Autodesk Inventor part; units mm, degrees
ref_plane "YZ Plane" through (0, 0, 0) normal (1, 0, 0) x (0, 1, 0)
ref_plane "XZ Plane" through (0, 0, 0) normal (0, 1, 0) x (-1, 0, 0)
sketch "Sketch1" plane through (0, 0, 0) normal (0, 1, 0) x (-1, 0, 0)
  circle A0 centre (0, 0) radius 75
  dimension "d0" = 150
extrude "Extrusion1" add sketch "Sketch1" along normal blind 200
sketch "Sketch2" plane through (0, 200, 0) normal (0, 1, 0) x (1, 0, 0)
  circle A0 centre (0, 0) radius 75
  circle A1 centre (0, 0) radius 70
  dimension "d3" = 5
extrude "Extrusion2" cut sketch "Sketch2" against normal blind 195 contours A1
ref_plane "Work Plane1" through (0, 0, -75) normal (0, 0, 1) x (1, 0, 0)
sketch "Sketch4" plane through (0, 0, -75) normal (0, 0, 1) x (1, 0, 0)
  line L0 (15, 185) -> (-15, 185)
  line L1 (-15, 185) -> (-15, 155)
  line L2 (-15, 155) -> (15, 155)
  line L3 (15, 155) -> (15, 185)
  line L4 (15, 185) -> (-15, 155) construction
  line L5 (-15, 185) -> (15, 155) construction
  line L6 (75, 200) -> (-75, 200) construction
  line L7 (0, 170) -> (0, 200) construction
  circle A0 centre (0, 170) radius 11.05
  point P0 (0, 0)
  dimension "d8" = 30
  dimension "d9" = 30
  dimension "d10" = 30
  dimension "d15" = 22.1
extrude "Extrusion3" add sketch "Sketch4" along normal blind 3 and the other way blind 10
mirror "Mirror1" about plane through (0, 0, 0) normal (0, 0, 1) of "Extrusion3"
sketch "Sketch5" plane through (0, 0, 0) normal (0, -1, 0) x (1, 0, 0)
  line L0 (15, -4) -> (-15, -4)
  line L1 (-15, -4) -> (-15, 4)
  line L2 (-15, 4) -> (15, 4)
  line L3 (15, 4) -> (15, -4)
  line L4 (15, -4) -> (-15, 4) construction
  line L5 (-15, -4) -> (15, 4) construction
  circle A0 centre (0, 0) radius 75
  dimension "d27" = 30
  dimension "d28" = 8
extrude "Extrusion4" add sketch "Sketch5" along normal blind 35 contours L0 L1 L2 L3
sketch "Sketch7" plane through (-15, 0, 4) normal (0, 0, 1) x (1, 0, 0)
  circle A0 centre (15, -20) radius 11.05
  line L0 (0, 0) -> (0, -35)
  line L1 (30, -35) -> (0, -35)
  point P0 (15, 0)
  dimension "d29" = 22.1
  dimension "d30" = 15
  dimension "d31" = 15
extrude "Extrusion6" cut sketch "Sketch7" against normal up to surface (8 mm away)
sketch "Sketch8" plane through (-15, 0, 4) normal (0, 0, 1) x (1, 0, 0)
  circle A0 centre (15, -20) radius 11.05
  line L0 (0, 0) -> (30, 0)
  line L1 (0, 0) -> (0, -35)
  line L2 (30, -35) -> (0, -35)
  line L3 (30, 0) -> (30, -35)
  arc A1 (0, -20) -> (30, -20) centre (15, -18.2651) ccw
  line L4 (0, -20) -> (30, -20)
  line L5 (30, -20) -> (30, -35)
  line L6 (30, -35) -> (0, -35)
  line L7 (0, -35) -> (0, -20)
  dimension "d37" = 15.1
extrude "Extrusion8" cut sketch "Sketch8" against normal blind 35 contours L3 L2 L1 A1
sketch "Sketch9" plane through (15, 155, 73.4847) normal (1, 0, 0) x (0, 0, -1)
  line L0 (-11.5153, 30) -> (0, 30)
  line L1 (0, 30) -> (-20, 30)
  line L2 (-20, 30) -> (-20, 20)
  line L3 (-20, 20) -> (0, 20)
  line L4 (0, 20) -> (0, 30)
  point P0 (73.4847, -155)
  dimension "d40" = 20
  dimension "d41" = 10
extrude "Extrusion9" add sketch "Sketch9" along normal blind 10
mirror "Mirror2" about plane through (0, 0, 0) normal (0, 0, 1) of "Extrusion9"
chamfer "Chamfer1" distance 3 angle 45 2 edges at (15, 175, 89.2423) (15, 175, -89.2423)
ref_plane "Work Plane2" through (0, 0, 75) normal (0, 0, 1) x (1, 0, 0)
sketch "Sketch10" plane through (0, 0, 75) normal (0, 0, 1) x (1, 0, 0)
  line L0 (2.6, 190.2) -> (-2.6, 190.2)
  line L1 (-2.6, 190.2) -> (-2.6, 185)
  line L2 (-2.6, 185) -> (2.6, 185)
  line L3 (2.6, 185) -> (2.6, 190.2)
  line L4 (-15, 155) -> (-15, 185)
  line L5 (15, 155) -> (-15, 155)
  line L6 (15, 175) -> (15, 155)
  line L7 (15, 175) -> (18, 175)
  line L8 (18, 175) -> (15, 178)
  line L9 (15, 185) -> (15, 178)
  line L10 (-15, 185) -> (15, 185)
  circle A0 centre (0, 170) radius 11.05
  line L11 (15, 185) -> (-15, 185) construction
  line L12 (0, 185) -> (0, 170) construction
  line L13 (-70, 200) -> (70, 200)
  line L14 (-2.6, 185) -> (-7.8, 185)
  line L15 (-7.8, 185) -> (-7.8, 200)
  line L16 (-7.8, 200) -> (-2.6, 200)
  line L17 (-2.6, 200) -> (-2.6, 185)
  point P0 (0, 0)
  dimension "d50" = 5.2
  dimension "d51" = 5.2
  dimension "d52" = 5.2
extrude "Extrusion10" cut sketch "Sketch10" against normal up to surface contours L3 L2 L1 L0 | L1 L10 L15 L13 L17
pattern_circular "Circular Pattern1" count 4 over 360 about axis through (0, 200, 0) along (0, -1, 0) of "Extrusion10"
sketch "Sketch11" plane through (0, 0, 75) normal (0, 0, 1) x (1, 0, 0)
  line L0 (-70, 5) -> (70, 5)
  line L1 (69.5641, 200) -> (69.5641, 185)
  line L2 (69.5641, 185) -> (69.9517, 185)
  line L3 (69.9517, 185) -> (69.9517, 190.2)
  line L4 (69.9517, 190.2) -> (69.9517, 190.2)
  line L5 (69.9517, 190.2) -> (69.9517, 200)
  line L6 (7.8, 200) -> (69.9517, 200)
  line L7 (7.8, 200) -> (7.8, 185)
  line L8 (7.8, 185) -> (-2.6, 185)
  line L9 (-2.6, 185) -> (-2.6, 190.2)
  line L10 (-2.6, 190.2) -> (2.6, 190.2)
  line L11 (2.6, 190.2) -> (2.6, 200)
  line L12 (-69.5641, 200) -> (2.6, 200)
  line L13 (-69.5641, 200) -> (-69.5641, 185)
  line L14 (-69.5641, 185) -> (-69.9517, 185)
  line L15 (-69.9517, 185) -> (-69.9517, 190.2)
  line L16 (-69.9517, 190.2) -> (-69.9517, 190.2)
  line L17 (-69.9517, 190.2) -> (-69.9517, 200)
  line L18 (-7.8, 200) -> (-69.9517, 200)
  line L19 (-7.8, 200) -> (-7.8, 185)
  line L20 (-7.8, 185) -> (2.6, 185)
  line L21 (2.6, 185) -> (2.6, 190.2)
  line L22 (2.6, 190.2) -> (-2.6, 190.2)
  line L23 (-2.6, 190.2) -> (-2.6, 200)
  line L24 (69.5641, 200) -> (-2.6, 200)
  line L25 (-17.8, 200) -> (-7.8, 200)
  line L26 (-7.8, 200) -> (-7.8, 195)
  line L27 (-7.8, 195) -> (-17.8, 195)
  line L28 (-17.8, 195) -> (-17.8, 200)
  point P0 (0, 0)
  dimension "d58" = 10
  dimension "d59" = 5
extrude "Extrusion11" cut sketch "Sketch11" against normal up to surface contours L19 L27 L28 L12
pattern_circular "Circular Pattern2" count 2 over 360 about axis through (0, 0, 0) along (0, 1, 0) of "Extrusion11"
properties part number "main_body"
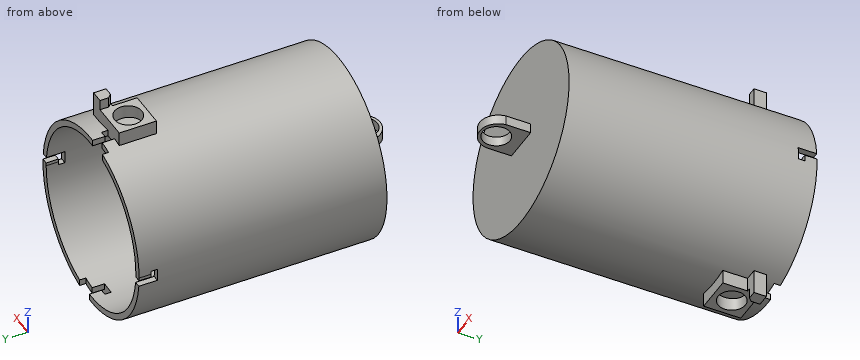
Design review of the part built by this model. Coordinates are the model's own, in mm. Coordinates: 2 decimals unless noted, no trailing zeros. Write each loop counter-clockwise with the first axis right and the second up, starting at its lowest first coordinate (ties: lowest second). Pieces come first, ordered by that corner, then holes. Notation, with made-up numbers: (-16, -12.75) - (-8, -12.75) arc R12 cw to (-8, 6.25) - close; hole circle Ø9 at (30.5, 47). An arc over 180 degrees is marked (long way). One line per item, written item: value.
1) To check wall thickness, follow probe 1 along X at (y, z) = (49.5, 1); probe 2 along X at (y, z) = (168, -8); probe 3 along Y at (x, z) = (0, 77). State the ranges of each line that lie inside material, in increasing order.
Answer sheet:
probe 1: x = -74.99 to -69.99, 69.99 to 74.99
probe 2: x = -74.57 to -69.54, 69.54 to 74.57
probe 3: y = 155 to 158.95, 181.05 to 185
2) Add section D-D (z = -18.5). State the section outline as (x, y) points, plus the area to 3 significant figures.
Answer sheet:
outline: (-72.68, 0) - (72.68, 0) - (72.68, 200) - (67.51, 200) - (67.51, 5) - (-67.51, 5) - (-67.51, 200) - (-72.68, 200) - close
area: 2,740 mm2
3) Insertion check: pin 1 (12 mm diameter, centred on x = -19, z = -53.5, fed in from +Y); pin 2 (1 mm diameter, centred on x = 11, y = 42, fed in from +Z); pin 3 (4 mm diameter, centred on y = 47.5, z = 56.5, fed in from -X). Each pin has a flat end and moves straight along its axis. Give the tip position at first contact, or say it passes through.
Answer sheet:
pin 1: stops at y = 5
pin 2: stops at z = 74.26
pin 3: stops at x = -51.52
4) Add section C-C (x = 65). State the section outline as (y, z) points.
Answer sheet:
outline: (0, -37.42) - (200, -37.42) - (200, -25.98) - (5, -25.98) - (5, 25.98) - (200, 25.98) - (200, 37.42) - (0, 37.42) - close
5) Add section A-A (y = 170). State the section outline as (x, z) points.
Answer sheet:
outline: (-15, -85) - (-11.05, -85) - (-11.05, -74.18) arc R75 ccw to (11.05, -74.18) - (11.05, -85) - (15, -85) - (15, -73.48) arc R75 ccw to (15, 73.48) - (15, 85) - (11.05, 85) - (11.05, 74.18) arc R75 ccw to (-11.05, 74.18) - (-11.05, 85) - (-15, 85) - (-15, 73.48) arc R75 ccw to (-15, -73.48) - close; hole circle Ø140 at (0, 0)
6) Add section B-B (z = -79). State the section outline as (x, y) points.
Answer sheet:
outline: (-15, 155) - (15, 155) - (15, 175) - (25, 175) - (25, 185) - (-15, 185) - close; hole circle Ø22.1 at (0, 170)
